Geometry check sheet. Reference: the model listing, model coordinates, mm. A direction names the side the tool comes from. Round coordinates to 2 decimals unless told otherwise and drop trailing zeros. Write each loop counter-clockwise with the first axis right and the second up, starting at its lowest first coordinate (ties: lowest second). Pieces come first, ordered by that corner, then holes. Notation, with made-up numbers: M 41.5,41 L 57.5,41 A17 ccw 57.5,69 Z; hole C -34.75,83.5 d3. An arc over 180 degrees is marked long. Use a Markdown table: item, result.
Autodesk Inventor part; units mm, degrees
ref_plane "YZ Plane" through (0, 0, 0) normal (1, 0, 0) x (0, 1, 0)
ref_plane "XZ Plane" through (0, 0, 0) normal (0, 1, 0) x (-1, 0, 0)
ref_plane "XY Plane" through (0, 0, 0) normal (0, 0, 1) x (1, 0, 0)
sketch "草圖1" plane through (0, 0, 0) normal (0, 1, 0) x (-1, 0, 0)
  line L0 (0, 0) -> (-60, 0)
  line L1 (-60, 0) -> (-60, -70)
  line L2 (-60, -70) -> (0, -70)
  line L3 (0, -70) -> (0, 0)
  dimension "d0" = 60
  dimension "d1" = 70
extrude "平板1" add sketch "草圖1" along normal blind 2
sketch "草圖2" plane through (2, 0, 0) normal (-1, 0, 0) x (0, -1, 0)
  line L0 (0, -70) -> (0, 0)
  line L1 (0, 0) -> (-22.5, 0)
  line L2 (-22.5, 0) -> (-22.5, -70)
  line L3 (-22.5, -70) -> (0, -70)
edge flange "凸緣1" height 22.5 angle 90 thickness 2 bend radius 0 thickness toward (-1, 0, 0) relief straight relief width 2 relief depth 1 edges at (0, 2, -35) wall of the first edge with corners at (2, 0, -70) (2, 0, 0) (2, 22.5, 0) (2, 22.5, -70)
bend "折彎1"
corner "轉角1"
sketch "草圖3" plane through (58, 0, -70) normal (1, 0, 0) x (0, 1, 0)
  line L0 (0, 70) -> (0, 0)
  line L1 (0, 0) -> (22.5, 0)
  line L2 (22.5, 0) -> (22.5, 70)
  line L3 (22.5, 70) -> (0, 70)
edge flange "凸緣2" height 22.5 angle 90 thickness 2 bend radius 0 thickness toward (1, 0, 0) relief straight relief width 2 relief depth 1 edges at (60, 2, -35) wall of the first edge with corners at (58, 0, 0) (58, 0, -70) (58, 22.5, -70) (58, 22.5, 0)
bend "折彎2"
corner "轉角2"
chamfer "轉角倒角1" distance 5 angle 45 4 edges at (1, 22.5, -70) (1, 22.5, 0) (59, 22.5, -70) (59, 22.5, 0)
sketch "草圖4" plane through (60, 2.001, 0) normal (1, 0, 0) x (0, 0, -1)
  line L0 (15, 11.999) -> (55, 11.999)
  line L1 (70, -2.001) -> (0, -2.001)
  line L2 (0, 0) -> (0, 15.499)
  dimension "d26" = 40
  dimension "d27" = 14
  dimension "d28" = 15
hole "孔1" at (60, 14, -15) at (60, 14, -55) direction (-1, 0, 0) diameter 5 depth 80 tip angle 118
equation "\"d3\" = 折彎離隙寬度"
equation "\"d4\" = 折彎離隙深度"
equation "\"d5\" = 最小剩餘"
equation "\"d6\" = 折彎半徑"
equation "\"d10\" = 轉角離隙大小"
equation "\"d11\" = 間隙大小"
equation "\"d12\" = Jacobi半徑大小"
equation "\"d13\" = 折彎離隙寬度"
equation "\"d14\" = 折彎離隙深度"
equation "\"d15\" = 最小剩餘"
equation "\"d16\" = 折彎半徑"
equation "\"d20\" = 轉角離隙大小"
equation "\"d21\" = 間隙大小"
equation "\"d22\" = Jacobi半徑大小"
equation "\"折彎半徑\" = 厚度"
equation "\"折彎離隙寬度\" = 厚度"
equation "\"折彎離隙深度\" = 0.5 * 厚度"
equation "\"轉角離隙大小\" = 4 * 厚度"
equation "\"最小剩餘\" = 2 * 厚度"
equation "\"轉移半徑\" = 折彎半徑"
equation "\"Jacobi半徑大小\" = 厚度"
equation "\"間隙大小\" = 厚度"
equation "\"d2\" = 折彎半徑"
properties part number "4-4"
Item 1: Cross-section at A-A, the plane y = 14. Record the cut outline in (x, z).
Outcome:
| item | result |
|---|---|
| outline | M 0,-70 L 2,-70 L 2,-57.5 L 0,-57.5 Z; M 0,-52.5 L 2,-52.5 L 2,-17.5 L 0,-17.5 Z; M 0,-12.5 L 2,-12.5 L 2,0 L 0,0 Z; M 58,-70 L 60,-70 L 60,-57.5 L 58,-57.5 Z; M 58,-52.5 L 60,-52.5 L 60,-17.5 L 58,-17.5 Z; M 58,-12.5 L 60,-12.5 L 60,0 L 58,0 Z |
Item 2: Mould release check, pull along Y, two halves, no side actions. Record for faces 3 (the face through (0, 12, -35)), 4 (the face through (1, 20, -2.5)), 5 (the face through (1, 13.9, -12.5)): +Y half, -Y half, draft (parallel to the pull), parting line (faces both ways), or undercut.
Outcome:
| item | result |
|---|---|
| face 3 | draft |
| face 4 | +Y half |
| face 5 | undercut |
Item 3: Go/stop test with flat-tipped pins: pin 1 (3 mm diameter, centred on x = 48.5, z = -52.5, fed in from -Y); pin 2 (4 mm diameter, centred on y = 14, z = -55, fed in from +X); pin 3 (12 mm diameter, centred on x = 21.5, z = -61, fed in from +Y). Record where each tip stops, or that it passes through.
Outcome:
| item | result |
|---|---|
| pin 1 | stops at y = 0 |
| pin 2 | passes through |
| pin 3 | stops at y = 2 |
Item 4: Cross-section at B-B, the plane z = -55. Record the cut outline in (x, y).
Outcome:
| item | result |
|---|---|
| outline | M 0,2 A2 ccw 2,0 L 58,0 A2 ccw 60,2 L 60,11.5 L 58,11.5 L 58,2 L 2,2 L 2,11.5 L 0,11.5 Z; M 0,16.5 L 2,16.5 L 2,22.5 L 0,22.5 Z; M 58,16.5 L 60,16.5 L 60,22.5 L 58,22.5 Z |
Item 5: Cross-section at C-C, the plane y = 5.5. Record the cut outline in (x, z), and give its area (3 significant figures).
Outcome:
| item | result |
|---|---|
| outline | M 0,-70 L 2,-70 L 2,0 L 0,0 Z; M 58,-70 L 60,-70 L 60,0 L 58,0 Z |
| area | 280 mm2 |
Item 6: Material ranges on line 1 along Z through (x, y) = (0.6, 14); line 2 along X through (y, z) = (9.75, -11.5); line 3 along Y through (x, z) = (3, -5.5), recorded low to high. Write a range as from..to.
Outcome:
| item | result |
|---|---|
| line 1 | z = -70..-57.5, -52.5..-17.5, -12.5..0 |
| line 2 | x = 0..2, 58..60 |
| line 3 | y = 0..2 |
Item 7: Cross-section at D-D, the plane z = -8. Record the cut outline in (x, y), and give its area (3 significant figures).
Outcome:
| item | result |
|---|---|
| outline | M 0,2 A2 ccw 2,0 L 58,0 A2 ccw 60,2 L 60,22.5 L 58,22.5 L 58,2 L 2,2 L 2,22.5 L 0,22.5 Z |
| area | 200 mm2 |
Item 8: Access from +Z, -Z, +X, -X, +Y, -Y to the whole of each face (thin tool, end or side, straight path). Record for faces 1 (the face through (59, 22.5, -35)), 2 (the face through (58, 12, -35)).
Outcome:
| item | result |
|---|---|
| face 1 | +Z, -Z, +X, -X, +Y |
| face 2 | +Z, -Z, +Y |
